Model file for the job. Use its own axes, mm. Round coordinates to 2 decimals unless told otherwise and drop trailing zeros. Order: outer loops, then holes, each group sorted by start corner. A loop starts at its lowest first (then second) coordinate and runs counter-clockwise, first axis right, second up. Notation, with made-up numbers: (-31, -20.75) -> (12, -20.75) arc R34 ccw to (12, 17.25) -> close; hole circle Ø1 at (-38.75, -6). An arc over 180 degrees is marked (long way). Put each result on its own line as item: value. Start each with the question number.
Q1. Pull direction Y, two halves, no side cores. Call faces 1 (the face through (2, -2, 0)), 2 (the face through (-2.17, -9.76, 0.99)), 3 (the face through (-0.238, 6.926, 0.986)): released by +Y, released by -Y, zero draft, split by the parting line, or undercut.
Q2. Cut at A-A, the plane x = 8. List the corners of the cut face in (y, z).
Q3. Cut at B-B, the plane y = 0. List the corners of the cut face in (x, z).
Q4. Probe L1, parallel to Y at x = 0, z = 1.4; L2, parallel to X at y = -0.5, z = 0.25; L3, parallel to X at y = 0.25, z = 1.2. List the from-to ranges inside material, lowest first.
Q5. Cut at D-D, the plane z = 1.2. List the corners of the cut face in (x, y), and give its area (3 significant figures).
Q6. Flat gauge pins, fed straight in: P1, Ø3.5, axis at x = 8, y = 0, coming from the -Z side; P2, Ø1, axis at y = 2.5, z = 0.5, coming from the +X side; P3, Ø1, axis at x = 3, z = 0, coming from the +Y side. Where does each tip first touch, or does it go through?
from build123d import *

# Parameters (mm, degrees)
HORN_PLATE_ENVELOPE_PROFILE_R           = 10
HORN_PLATE_ENVELOPE_PROFILE_R_2         = 2.55
HORN_PLATE_ENVELOPE_DEPTH               = 2
NOMINAL_HORN_ATTACHMENT_HOLES_START     = -50
NOMINAL_HORN_ATTACHMENT_HOLES_PROFILE_R = 1.1
NOMINAL_HORN_ATTACHMENT_HOLES_DEPTH     = 65.282856857


with BuildPart() as part:
    # Horn_plate_envelope_profile → Horn_plate_envelope (new body)
    with BuildSketch(Plane.XY):
        Circle(HORN_PLATE_ENVELOPE_PROFILE_R)
        Circle(HORN_PLATE_ENVELOPE_PROFILE_R_2, mode=Mode.SUBTRACT)
    extrude(amount=HORN_PLATE_ENVELOPE_DEPTH)

    # Nominal_horn_attachment_holes_profile → Nominal_horn_attachment_holes (cut, through all)
    with BuildSketch(Plane.XY.offset(NOMINAL_HORN_ATTACHMENT_HOLES_START)):
        with Locations((-8, 0)):
            Circle(NOMINAL_HORN_ATTACHMENT_HOLES_PROFILE_R)
        with Locations((8, 0)):
            Circle(NOMINAL_HORN_ATTACHMENT_HOLES_PROFILE_R)
        with Locations((0, -8)):
            Circle(NOMINAL_HORN_ATTACHMENT_HOLES_PROFILE_R)
        with Locations((0, 8)):
            Circle(NOMINAL_HORN_ATTACHMENT_HOLES_PROFILE_R)
    extrude(amount=NOMINAL_HORN_ATTACHMENT_HOLES_DEPTH, mode=Mode.SUBTRACT)


solid = part.part
Ans:
1. face 1: zero draft
1. face 2: split by the parting line
1. face 3: undercut
2. outline: (-6, 0) -> (-1.1, 0) -> (-1.1, 2) -> (-6, 2) -> close; (1.1, 0) -> (6, 0) -> (6, 2) -> (1.1, 2) -> close
3. outline: (-10, 0) -> (-9.1, 0) -> (-9.1, 2) -> (-10, 2) -> close; (-6.9, 0) -> (-2.55, 0) -> (-2.55, 2) -> (-6.9, 2) -> close; (2.55, 0) -> (6.9, 0) -> (6.9, 2) -> (2.55, 2) -> close; (9.1, 0) -> (10, 0) -> (10, 2) -> (9.1, 2) -> close
4. L1: y = -10 to -9.1, -6.9 to -2.55, 2.55 to 6.9, 9.1 to 10
4. L2: x = -9.99 to -8.98, -7.02 to -2.5, 2.5 to 7.02, 8.98 to 9.99
4. L3: x = -10 to -9.07, -6.93 to -2.54, 2.54 to 6.93, 9.07 to 10
5. outline: circle Ø20 at (0, 0); hole circle Ø2.2 at (-8, 0); hole circle Ø5.1 at (0, 0); hole circle Ø2.2 at (0, -8); hole circle Ø2.2 at (0, 8); hole circle Ø2.2 at (8, 0)
5. area: 279 mm^2
6. P1: stops at z = 0
6. P2: stops at x = 9.8
6. P3: stops at y = 9.68
